Input: part model. Units: mm. Frame: model coordinates. A direction names the side the tool comes from. Coordinates: 2 decimals unless noted, no trailing zeros. Order: outer loops, then holes, each group sorted by start corner. A loop starts at its lowest first (then second) coordinate and runs counter-clockwise, first axis right, second up. Notation, with made-up numbers: M -2.75,16.5 L 14.25,16.5 A24 ccw 14.25,50.5 Z; hole C 89,-14.5 d4. An arc over 180 degrees is marked long. One line per item, written item: value.
```python
from build123d import *

# Parameters (mm, degrees)
F0_W           = 76.2
F0_H           = 76.2
F1_DEPTH       = 19.05
F3_DEPTH       = 25.4
F5_D           = 4.699
F5_CSINK_D     = 8.255
F5_CSINK_ANGLE = 90
F6_F1_R        = 3.175
F6_F2_R        = 3.175


with BuildPart() as f1:
    # F0 (on Front) → F1 (new body)
    with BuildSketch(Plane.XZ):
        Rectangle(F0_W, F0_H)
    extrude(amount=F1_DEPTH)

    # F2 (on face) → F3 (join)
    with BuildSketch(Plane.XZ.offset(19.05)):
        with BuildLine():
            ThreePointArc((13.462, 0), (0, -13.462), (-13.462, 0))
            Line((-13.462, 0), (-13.462, 15.875))
            Line((-13.462, 15.875), (-22.987, 15.875))
            Line((-22.987, 15.875), (-22.987, 0))
            ThreePointArc((-22.987, 0), (0, -22.987), (22.987, 0))
            Line((22.987, 0), (22.987, 15.875))
            Line((22.987, 15.875), (13.462, 15.875))
            Line((13.462, 15.875), (13.462, 0))
        make_face()
    extrude(amount=F3_DEPTH)

    # F5 (through all)
    with Locations(Plane.XZ.offset(19.05)):
        with Locations((-28.575, 28.575), (28.575, 28.575), (28.575, -28.575), (-28.575, -28.575)):
            CounterSinkHole(F5_D / 2, F5_CSINK_D / 2, counter_sink_angle=F5_CSINK_ANGLE)

    # F6: fillet of radius 3.175 on 23 edges, made by hand

    # F6_f1
    f6_f1_edges = [f1.edges().sort_by_distance(p)[0] for p in [
        (-38.1, -19.05, 0),
        (0, -19.05, 38.1),
        (38.1, -19.05, 0),
        (0, -19.05, -38.1),
        (0, -44.45, -22.987),
        (38.1, -9.525, -38.1),
        (38.1, -9.525, 38.1),
        (-38.1, -9.525, 38.1),
        (-38.1, -9.525, -38.1),
        (-13.462, -31.75, 15.875),
        (13.462, -31.75, 15.875),
        (22.987, -31.75, 15.875),
        (-22.987, -31.75, 15.875),
        (-18.2245, -44.45, 15.875),
        (18.2245, -44.45, 15.875),
        (22.987, -44.45, 7.9375),
        (-22.987, -44.45, 7.9375),
    ]]
    fillet(f6_f1_edges, radius=F6_F1_R)

    # F6_f2
    f6_f2_edges = [f1.edges().sort_by_distance(p)[0] for p in [
        (0, -19.05, -22.987),
        (0, -19.05, -13.462),
        (13.462, -19.05, 6.35),
        (-13.462, -19.05, 6.35),
        (22.987, -19.05, 6.35),
        (-22.987, -19.05, 6.35),
        (-22.0570640303, -19.05, 14.9450640303),
        (22.0570640303, -19.05, 14.9450640303),
        (-14.3919359697, -19.05, 14.9450640303),
        (14.3919359697, -19.05, 14.9450640303),
    ]]
    fillet(f6_f2_edges, radius=F6_F2_R)


solid = f1.part
```
(1) Cut plane A-A on x = 0. Output: boundary loops of the cut face in (y, z) (3 decimals).
Data:
outline: M -44.45,-19.812 A3.175 ccw -41.275,-22.987 L -22.225,-22.987 A3.175 cw -19.05,-26.162 L -19.05,-34.925 A3.175 ccw -15.875,-38.1 L 0,-38.1 L 0,38.1 L -15.875,38.1 A3.175 ccw -19.05,34.925 L -19.05,-10.287 A3.175 cw -22.225,-13.462 L -44.45,-13.462 Z
(2) Draft query along X for faces 1 (the cylindrical face through (23.942, -19.955, 6.439)), 2 (the cylindrical face through (29.08, -8.52, 26.28)), 3 (the cylindrical face through (-0.51, -31.62, -22.98)). Return one class per face: released by +X, released by -X, zero draft, split by the parting line, or undercut.
Data:
face 1: released by +X
face 2: undercut
face 3: split by the parting line
(3) Access query for faces 4 (the flat face through (18, -32, 15.875)), 5 (the flat face through (-13.462, -33, 6)), 6 (the flat face through (22.987, -32, 6)). Directions: +Z, -Z, +X, -X, +Y, -Y. A direction counts if a zero-diameter tool reaches every point of the face in a straight line with its end or side. Return the directions, or none.
Data:
face 4: +Z, +X, -X, -Y
face 5: +Z, -Y
face 6: +Z, -Z, +X, -Y
(4) First-contact query: pin 1 (6 mm diameter, centred on x = 28.575, z = 28.575, fed in from -Y); pin 2 (14 mm diameter, centred on y = -29.5, z = 9, fed in from +X); pin 3 (1 mm diameter, centred on x = 18.5, y = -35.5, fed in from +Z) (3 decimals). Flat tips, straight axial feed; report the tip coordinate or a pass-through.
Data:
pin 1: stops at y = -17.92
pin 2: stops at x = 22.99
pin 3: stops at z = 15.875
(5) Cut plane B-B on y = -36.5. Output: boundary loops of the cut face in (x, z) (3 decimals), plus the area to 3 significant figures.
Data:
outline: M -22.987,0 A22.987 ccw 22.987,0 L 22.987,12.7 A3.175 ccw 19.812,15.875 L 16.637,15.875 A3.175 ccw 13.462,12.7 L 13.462,0 A13.462 cw -13.462,0 L -13.462,12.7 A3.175 ccw -16.637,15.875 L -19.812,15.875 A3.175 ccw -22.987,12.7 Z
area: 839 mm2
(6) Ray query, line 1 (Y direction, x = 33, z = -4); line 2 (X direction, y = -24.5, z = -11); line 3 (X direction, y = -7.5, z = -26.5). Return the intervals inside material, ascending. Write a range as from..to.
Data:
line 1: y = -19.05..0
line 2: x = -20.18..-7.76, 7.76..20.18
line 3: x = -38.1..-29.68, -27.47..27.47, 29.68..38.1
